from build123d import *

# Parameters (mm, degrees)
F1_DEPTH    = 5
F2_T1_DEPTH = 28.770290161


# Not quite as in the source:
# - a fillet or chamfer that OpenCascade refuses, or shapes differently, is made with other operations: its cross-section is extruded or revolved along the edge and cut away or added


with BuildPart() as f1:
    # F0 (on Top) → F1 (new body)
    with BuildSketch(Plane.XY):
        Polygon((-10, 0), (0, 0), (10, 0), (23.8918542134, 78.784620241), (31.8918542134, 78.784620241), (31.8918542134, 81.784620241), (19.7553724367, 81.784620241), (19.7553724367, 78.3334689187), (7.6, 9.3969262079), (2.6, 9.3969262079), (2.6, 4.3969262079), (0, 4.3969262079), (-2.6, 4.3969262079), (-2.6, 9.3969262079), (-7.6, 9.3969262079), (-19.7553724367, 78.3334689187), (-19.7553724367, 81.784620241), (-31.8918542134, 81.784620241), (-31.8918542134, 78.784620241), (-23.8918542134, 78.784620241), align=None)
    extrude(amount=F1_DEPTH)

    # F2: fillet of radius 5 on 2 edges, made by hand

    # F2_s2 → F2_t1 (cut)
    with BuildSketch(Plane.XY.offset(-11.8851450805)):
        with BuildLine():
            ThreePointArc((-24.5094304689, 81.784620241), (-21.5721054433, 80.8308680948), (-19.7553724367, 78.3334689187))
            Line((-19.7553724367, 78.3334689187), (-19.7553724367, 81.784620241))
            Line((-19.7553724367, 81.784620241), (-24.5094304689, 81.784620241))
        make_face()
        with BuildLine():
            ThreePointArc((19.7553724367, 78.3334689187), (21.5721054433, 80.8308680948), (24.5094304689, 81.784620241))
            Line((24.5094304689, 81.784620241), (19.7553724367, 81.784620241))
            Line((19.7553724367, 81.784620241), (19.7553724367, 78.3334689187))
        make_face()
    extrude(amount=F2_T1_DEPTH, mode=Mode.SUBTRACT)


solid = f1.part
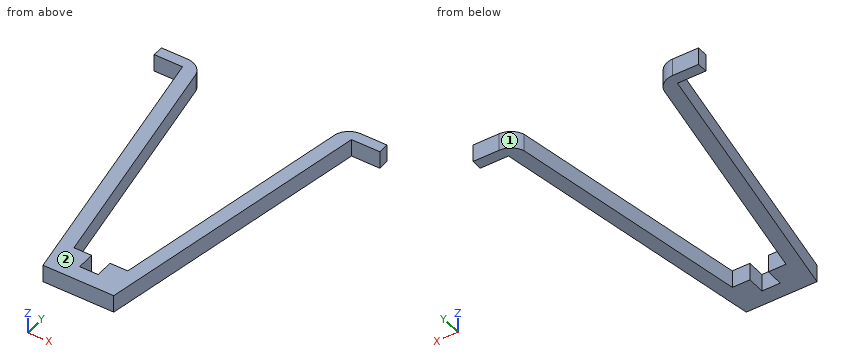
Here's how the part is built. I have some questions about the finished solid (model axes, mm). Face numbers are marked on the shaded views. Coordinates: 2 decimals unless noted, no trailing zeros. Order: outer loops, then holes, each group sorted by start corner. A loop starts at its lowest first (then second) coordinate and runs counter-clockwise, first axis right, second up. Notation, with made-up numbers: (-5.75, 61) - (35.25, 61) arc R23 ccw to (35.25, 78) - close; hole circle Ø2 at (53, -17). An arc over 180 degrees is marked (long way). Use CSV: the item, a comma, the result in double quotes. Start each with the question number.
1. Suppose I cut it at D-D on x = 1. List the corners of the cut face in (y, z) for me, then the cut area to 3 significant figures.
2. Suppose I cut it at B-B on z = 3. List the corners of the cut face in (x, y) for me.
3. Suppose I cut it at C-C on x = 25.5. List the corners of the cut face in (y, z) for me, then the cut area to 3 significant figures.
4. Please list where these lines run through material, in increasing order: line 1 (Y direction, x = 5.5, z = 1.8); line 2 (Y direction, x = 2.5, z = 3.1); line 3 (X direction, y = 13, z = 2.45). Write a range as from..to.
5. Suppose I cut it at A-A on y = 57. List the corners of the cut face in (x, z) for me, then the cut area to 3 significant figures.
6. If we mould it in two halves opening along X, with no side actions, what happens to the marked faces 1 and 2? For each: +X half, -X half, draft (parallel to the pull), parting line (faces both ways), or undercut.
7. I'm going to push flat-ended pins straight in: pin 1 (2.5 mm diameter, centred on x = 28.5, z = 3.5, fed in from -Y); pin 2 (2 mm diameter, centred on x = 14.5, y = 57, fed in from -Z); pin 3 (1.5 mm diameter, centred on x = 0, z = 3.5, fed in from +Y); pin 4 (1.5 mm diameter, centred on x = 6, z = 1.5, fed in from +Y). Where does each tip first touch, or does it pass through?
Output:
1,outline,"(0, 0) - (4.4, 0) - (4.4, 5) - (0, 5) - close"
1,area,"22.0 mm2"
2,outline,"(-31.89, 78.78) - (-23.89, 78.78) - (-10, 0) - (10, 0) - (23.89, 78.78) - (31.89, 78.78) - (31.89, 81.78) - (24.51, 81.78) arc R5 ccw to (19.76, 78.33) - (7.6, 9.4) - (2.6, 9.4) - (2.6, 4.4) - (-2.6, 4.4) - (-2.6, 9.4) - (-7.6, 9.4) - (-19.76, 78.33) arc R5 ccw to (-24.51, 81.78) - (-31.89, 81.78) - close"
3,outline,"(78.78, 0) - (81.78, 0) - (81.78, 5) - (78.78, 5) - close"
3,area,"15.0 mm2"
4,line 1,"y = 0..9.4"
4,line 2,"y = 0..4.4"
4,line 3,"x = -12.29..-8.24, 8.24..12.29"
5,outline,"(-20.05, 0) - (-15.99, 0) - (-15.99, 5) - (-20.05, 5) - close; (15.99, 0) - (20.05, 0) - (20.05, 5) - (15.99, 5) - close"
5,area,"40.6 mm2"
6,face 1,"undercut"
6,face 2,"draft"
7,pin 1,"stops at y = 78.78"
7,pin 2,"passes through"
7,pin 3,"stops at y = 4.4"
7,pin 4,"stops at y = 9.4"
